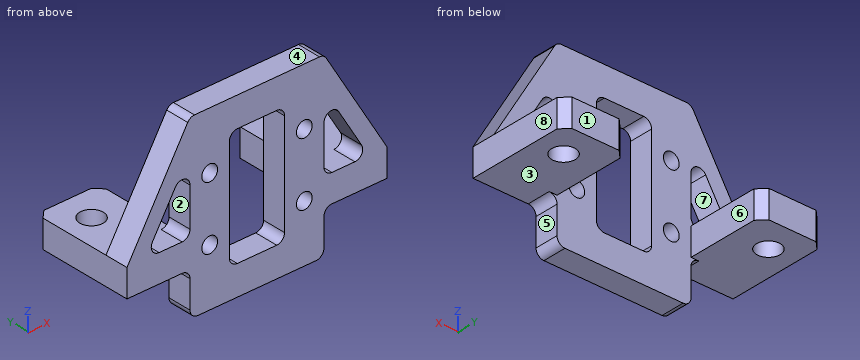
```python
from build123d import *

# Parameters (mm, degrees)
SKETCH_1_W          = 17
SKETCH_1_H          = 22.5
EXTRUDE_1_DEPTH     = 3
EXTRUDE_START       = 5.5
SKETCH_2_W          = 33
SKETCH_2_H          = 13
SKETCH_2_R          = 1.5
EXTRUDE_2_DEPTH     = 3.5
SKETCH_3_R          = 1
CUT_EXTRUDE_1_DEPTH = 24.828816588
SKETCH_4_W          = 17
SKETCH_4_H          = 3.5
CUT_EXTRUDE_2_DEPTH = 10
SKETCH_5_W          = 7
SKETCH_5_H          = 15
CUT_EXTRUDE_3_DEPTH = 23.334110683
EXTRUDE_3_DEPTH     = 3
FILLET_1_R          = 1
FILLET_2_R          = 1
CHAMFER_2_SIZE      = 1


with BuildPart() as part:
    # 草图1 → 凸台-拉伸1 (new body)
    with BuildSketch(Plane(origin=(0, 0, 0), x_dir=(1, 0, 0), z_dir=(0, 1, 0))):
        Rectangle(SKETCH_1_W, SKETCH_1_H)
    extrude(amount=EXTRUDE_1_DEPTH)

    # 草图2 → 凸台-拉伸2 (add)
    with BuildSketch(Plane.XY.offset(-11.25).offset(EXTRUDE_START)):
        with Locations((0, 6.5)):
            Rectangle(SKETCH_2_W, SKETCH_2_H)
        with Locations((-13, 9)):
            Circle(SKETCH_2_R, mode=Mode.SUBTRACT)
        with Locations(Location((13, 9, 0), (0, 0, 180))):
            Circle(SKETCH_2_R, mode=Mode.SUBTRACT)
    extrude(amount=EXTRUDE_2_DEPTH)

    # 草图3 → 切除-拉伸1 (cut, through all)
    with BuildSketch(Plane.XZ):
        with Locations(Location((6, -4, 0), (0, 0, 270))):
            Circle(SKETCH_3_R)
        with Locations(Location((-6, -4, 0), (0, 0, 270))):
            Circle(SKETCH_3_R)
        with Locations(Location((-6, 4, 0), (0, 0, 270))):
            Circle(SKETCH_3_R)
        with Locations(Location((6, 4, 0), (0, 0, 270))):
            Circle(SKETCH_3_R)
    extrude(amount=-CUT_EXTRUDE_1_DEPTH, mode=Mode.SUBTRACT)

    # 草图4 → 切除-拉伸2 (cut)
    with BuildSketch(Plane(origin=(0, 13, 0), x_dir=(1, 0, 0), z_dir=(0, 1, 0))):
        with Locations((0, 4)):
            Rectangle(SKETCH_4_W, SKETCH_4_H)
    extrude(amount=-CUT_EXTRUDE_2_DEPTH, mode=Mode.SUBTRACT)

    # 草图5 → 切除-拉伸3 (cut, through all)
    with BuildSketch(Plane(origin=(0, 3, 0), x_dir=(1, 0, 0), z_dir=(0, 1, 0))):
        Rectangle(SKETCH_5_W, SKETCH_5_H)
    extrude(amount=-CUT_EXTRUDE_3_DEPTH, mode=Mode.SUBTRACT)

    # 草图6 → 凸台-拉伸3 (add)
    with BuildSketch(Plane.XZ):
        Polygon((-16.5, -2.25), (-8.5, 11.25), (-8.5, 7.326911293), (-14.175206692, -2.25), align=None)
        Polygon((14.175206692, -2.25), (8.5, 7.326911293), (8.5, 11.25), (16.5, -2.25), align=None)
    extrude(amount=-EXTRUDE_3_DEPTH)

    # 圆角1
    fillet_1_edges = [part.edges().sort_by_distance(p)[0] for p in [
        (-8.5, 1.5, 7.326911293),
        (-14.175206692, 1.5, -2.25),
        (8.5, 1.5, 7.326911293),
        (14.175206692, 1.5, -2.25),
        (8.5, 1.5, -2.25),
        (-8.5, 1.5, -2.25),
        (3.5, 1.5, -7.5),
        (3.5, 1.5, 7.5),
        (-3.5, 1.5, 7.5),
        (-3.5, 1.5, -7.5),
    ]]
    fillet(fillet_1_edges, radius=FILLET_1_R)

    # 圆角2
    fillet_2_edges = [part.edges().sort_by_distance(p)[0] for p in [
        (8.5, 1.5, -5.75),
        (-8.5, 1.5, -5.75),
        (8.5, 1.5, 11.25),
        (-8.5, 1.5, 11.25),
        (-8.5, 1.5, -11.25),
        (8.5, 1.5, -11.25),
    ]]
    fillet(fillet_2_edges, radius=FILLET_2_R)

    # 倒角2
    chamfer_2_edges = [part.edges().sort_by_distance(p)[0] for p in [
        (16.5, 13, -4),
        (-16.5, 13, -4),
        (8.5, 13, -4),
        (-8.5, 13, -4),
    ]]
    chamfer(chamfer_2_edges, length=CHAMFER_2_SIZE)


solid = part.part
```
Could you check a few things on this model? Use its own coordinates, in mm. Face numbers are marked on the shaded views. A direction names the side the tool comes from. Round coordinates to 2 decimals unless told otherwise and drop trailing zeros. Loops run counter-clockwise (first coordinate to the right, second up) from the corner with the lowest first, then second, coordinate; pieces in that order, holes last. Notation, with made-up numbers: (74, 13.5) - (101, 13.5) arc R21 cw to (101, 22.5) - close; hole circle Ø10 at (-33, 50). An arc over 180 degrees is marked (long way). Use CSV: the item, a comma, the result in double quotes.
Item 1: If we section it at C-C on z = -0.25: List the corners of the cut face in (x, y) for me.
Here are the results:
outline,"(-15.31, 0) - (-12.99, 0) - (-12.99, 3) - (-15.31, 3) - close; (-8.5, 0) - (-3.5, 0) - (-3.5, 3) - (-8.5, 3) - close; (3.5, 0) - (8.5, 0) - (8.5, 3) - (3.5, 3) - close; (12.99, 0) - (15.31, 0) - (15.31, 3) - (12.99, 3) - close"
Item 2: If we mould it in two halves opening along Z, with no side actions, what happens to the marked faces 1, 2, 3 and 4? For each: pulls with the +Z half, pulls with the -Z half, needs draft (parallel to the pull), parting line crosses it, or undercut.
Here are the results:
face 1,"needs draft"
face 2,"undercut"
face 3,"pulls with the -Z half"
face 4,"pulls with the +Z half"
Item 3: I need wall thicknesses on L1, parallel to X at y = 0.85, z = -4; L2, parallel to Z at x = -2, y = 1; L3, parallel to X at y = 5, z = -5. Which ranges of each line are inside material? Lowest first, please. Write a range as [from, to].
Here are the results:
L1,"x = [-16.5, -7], [-5, -3.5], [3.5, 5], [7, 16.5]"
L2,"z = [-11.25, -7.5], [7.5, 11.25]"
L3,"x = [-16.5, -8.5], [8.5, 16.5]"
Item 4: For the marked faces 5, 6, 7 and 8, which set-ups out of +Z, -Z, +X, -X, +Y, -Y let a thin tool reach every point of the face, with its end or its side?
Here are the results:
face 5,"-Z, +X, +Y, -Y"
face 6,"+Z, -Z, +Y"
face 7,"+Y, -Y"
face 8,"+Z, -Z, +X, +Y, -Y"
Item 5: If we section it at D-D on x = 1: List the corners of the cut face in (y, z) for me.
Here are the results:
outline,"(0, -11.25) - (3, -11.25) - (3, -7.5) - (0, -7.5) - close; (0, 7.5) - (3, 7.5) - (3, 11.25) - (0, 11.25) - close"
Item 6: If we section it at B-B on x = -6: List the corners of the cut face in (y, z) for me, then the cut area to 3 significant figures.
Here are the results:
outline,"(0, -11.25) - (3, -11.25) - (3, -5) - (0, -5) - close; (0, -3) - (3, -3) - (3, 3) - (0, 3) - close; (0, 5) - (3, 5) - (3, 11.25) - (0, 11.25) - close"
area,"55.5 mm²"
Item 7: If we section it at A-A on y = 6.75: List the corners of the cut face in (x, z) for me.
Here are the results:
outline,"(-16.5, -5.75) - (-8.5, -5.75) - (-8.5, -2.25) - (-16.5, -2.25) - close; (8.5, -5.75) - (16.5, -5.75) - (16.5, -2.25) - (8.5, -2.25) - close"
Item 8: Will these pins go through, and if not, where does the flat tip stop? pin 1 (1.2 mm diameter, centred on x = 6, z = -4, fed in from +Y); pin 2 (2.5 mm diameter, centred on x = 6, z = 4, fed in from +Y); pin 3 (0.9 mm diameter, centred on y = 1, z = -8, fed in from +X); pin 4 (4 mm diameter, centred on x = -13, y = 9, fed in from +Z).
Here are the results:
pin 1,"passes through"
pin 2,"stops at y = 3"
pin 3,"stops at x = 8.5"
pin 4,"stops at z = -2.25"
